from build123d import *

# Parameters (mm, degrees)
SKETCH1_R           = 8.5
SKETCH1_R_2         = 4.05
BOSS_EXTRUDE1_DEPTH = 30
SKETCH2_R           = 15.7
SKETCH2_R_2         = 10.7
SKETCH2_R_3         = 8.5
SKETCH2_R_4         = 4.05
BOSS_EXTRUDE2_DEPTH = 5
BOSS_EXTRUDE3_START = 15
SKETCH3_R           = 15.7
SKETCH3_R_2         = 10.7
BOSS_EXTRUDE3_DEPTH = 15
FILLET1_R           = 1
CHAMFER1_SIZE       = 1
CHAMFER2_SIZE       = 1


with BuildPart() as part:
    # Sketch1 → Boss-Extrude1 (new body)
    with BuildSketch(Plane.XY):
        Circle(SKETCH1_R)
        Circle(SKETCH1_R_2, mode=Mode.SUBTRACT)
    extrude(amount=BOSS_EXTRUDE1_DEPTH)

    # Sketch2 → Boss-Extrude2 (add)
    # profile 1 of 3: a face of its own
    with BuildSketch(Plane.XY.offset(30)):
        Circle(SKETCH2_R)
        Circle(SKETCH2_R_2, mode=Mode.SUBTRACT)
    # profile 2 of 3: a face of its own
    with BuildSketch(Plane.XY.offset(30)):
        Circle(SKETCH2_R_2)
        Circle(SKETCH2_R_3, mode=Mode.SUBTRACT)
    # profile 3 of 3: a face of its own
    with BuildSketch(Plane.XY.offset(30)):
        Circle(SKETCH2_R_3)
        Circle(SKETCH2_R_4, mode=Mode.SUBTRACT)
    extrude(amount=BOSS_EXTRUDE2_DEPTH)

    # Sketch3 → Boss-Extrude3 (add)
    with BuildSketch(Plane(origin=(0, 0, 30), x_dir=(-1, 0, 0), z_dir=(0, 0, -1)).offset(BOSS_EXTRUDE3_START)):
        Circle(SKETCH3_R)
        Circle(SKETCH3_R_2, mode=Mode.SUBTRACT)
    extrude(amount=-BOSS_EXTRUDE3_DEPTH)

    # Fillet1
    fillet1_edges = [part.edges().sort_by_distance(p)[0] for p in [
        (10.7, 0, 30),
        (-8.5, 0, 30),
    ]]
    fillet(fillet1_edges, radius=FILLET1_R)

    # Chamfer1
    chamfer1_edges = [part.edges().sort_by_distance(p)[0] for p in [
        (10.7, 0, 15),
    ]]
    chamfer(chamfer1_edges, length=CHAMFER1_SIZE)

    # Chamfer2
    chamfer2_edges = [part.edges().sort_by_distance(p)[0] for p in [
        (-8.5, 0, 0),
        (-4.05, 0, 0),
    ]]
    chamfer(chamfer2_edges, length=CHAMFER2_SIZE)


solid = part.part
Here's how the part is built. I have some questions about the finished solid (model axes, mm). A direction names the side the tool comes from. Coordinates: 2 decimals unless noted, no trailing zeros. Write each loop counter-clockwise with the first axis right and the second up, starting at its lowest first coordinate (ties: lowest second). Pieces come first, ordered by that corner, then holes.
Item 1: I want a section at D-D on z = 4.5. Write out the boundary of the cut face in (x, y), and give its area (3 significant figures).
Item 2: If I drill on line 1 (Y direction, x = 0, z = 22.75); line 2 (Y direction, x = 0, z = 13); line 3 (Y direction, x = 0, z = 33), over which ranges is the centre line in solid material (lowest first)?
Item 3: On a 3-axis mill with a long thin cutter (end or side, diameter ignored), from which of +Z, -Z, +X, -X, +Y, -Y can I reach the whole of each face in a straight line? I mean faces 1 (the flat face through (0, 12, 15)), 2 (the flat face through (3, -3, 35)). Say none if no direction works.
Item 4: Will these pins go through, and if not, where does the flat tip stop? pin 1 (1 mm diameter, centred on x = 5, z = 11, fed in from -Y); pin 2 (10 mm diameter, centred on y = 7, z = 19, fed in from +X); pin 3 (1.5 mm diameter, centred on x = 12, y = -6.5, fed in from -Z).
Item 5: I want a section at A-A on y = 0. Write out the boundary of the cut face in (x, z), and give its area (3 significant figures).
Item 6: I want a section at B-B on z = 27. Write out the boundary of the cut face in (x, y).
Item 7: If we mould it in two halves opening along Y, with no side actions, what happens to faces 3 (the cylindrical face through (4.57, 7.167, 14.804)), 4 (the cylindrical face through (-0.878, -3.954, 17.762)), 5 (the flat face through (5, -2, 0))? For each: +Y half, -Y half, draft (parallel to the pull), parting line (faces both ways), or undercut.
Findings below:
1. outline: circle Ø17 at (0, 0); hole circle Ø8.1 at (0, 0)
1. area: 175 mm2
2. line 1: y = -15.7 to -10.7, -8.5 to -4.05, 4.05 to 8.5, 10.7 to 15.7
2. line 2: y = -8.5 to -4.05, 4.05 to 8.5
2. line 3: y = -15.7 to -4.05, 4.05 to 15.7
3. face 1: -Z
3. face 2: +Z, +X, -X, +Y, -Y
4. pin 1: stops at y = -7.21
4. pin 2: stops at x = 15.57
4. pin 3: stops at z = 15
5. outline: (-15.7, 15) - (-11.7, 15) - (-10.7, 16) - (-10.7, 29) arc R1 cw to (-9.7, 30) - (-9.5, 30) arc R1 cw to (-8.5, 29) - (-8.5, 1) - (-7.5, 0) - (-5.05, 0) - (-4.05, 1) - (-4.05, 35) - (-15.7, 35) - close; (4.05, 1) - (5.05, 0) - (7.5, 0) - (8.5, 1) - (8.5, 29) arc R1 cw to (9.5, 30) - (9.7, 30) arc R1 cw to (10.7, 29) - (10.7, 16) - (11.7, 15) - (15.7, 15) - (15.7, 35) - (4.05, 35) - close
5. area: 531 mm2
6. outline: circle Ø31.4 at (0, 0); circle Ø17 at (0, 0); hole circle Ø21.4 at (0, 0); hole circle Ø8.1 at (0, 0)
7. face 3: undercut
7. face 4: undercut
7. face 5: draft
